```python
from build123d import *

# Parameters (mm, degrees)
SKETCH_1_W          = 15
SKETCH_1_H          = 15
EXTRUDE_1_DEPTH     = 5
SKETCH_2_R          = 1.25
SKETCH_2_R_2        = 2.8
SKETCH_2_R_3        = 1.5
SKETCH_2_R_4        = 1
CUT_EXTRUDE_1_DEPTH = 5
FILLET_1_R          = 1.5
SKETCH_4_R          = 1.5
EXTRUDE_2_DEPTH     = 2
SKETCH_5_R          = 2
CUT_EXTRUDE_2_DEPTH = 5


with BuildPart() as part:
    # 草图1 → 凸台-拉伸1 (new body)
    with BuildSketch(Plane(origin=(0, 0, 0), x_dir=(1, 0, 0), z_dir=(0, 1, 0))):
        Polygon((25, 10), (-25, 10), (-25, 5), (-25, -10), (25, -10), align=None)
        with Locations((-32.5, -2.5)):
            Rectangle(SKETCH_1_W, SKETCH_1_H)
    extrude(amount=EXTRUDE_1_DEPTH)

    # 草图2 → 切除-拉伸1 (cut)
    with BuildSketch(Plane(origin=(0, 5, 0), x_dir=(1, 0, 0), z_dir=(0, 1, 0))):
        with Locations(Location((0, 0, 0), (0, 0, 270))):
            Circle(SKETCH_2_R)
        with Locations(Location((15, 0, 0), (0, 0, 270))):
            Circle(SKETCH_2_R_2)
        with Locations(Location((-15, 0, 0), (0, 0, 270))):
            Circle(SKETCH_2_R_2)
        with Locations(Location((15, 8, 0), (0, 0, 270))):
            Circle(SKETCH_2_R)
        with Locations(Location((23, 0, 0), (0, 0, 270))):
            Circle(SKETCH_2_R)
        with Locations(Location((-23, 0, 0), (0, 0, 270))):
            Circle(SKETCH_2_R)
        with Locations(Location((-15, 8, 0), (0, 0, 270))):
            Circle(SKETCH_2_R)
        with Locations(Location((-32.5, -2.5, 0), (0, 0, 270))):
            Circle(SKETCH_2_R_3)
        with Locations(Location((-27, -2.5, 0), (0, 0, 270))):
            Circle(SKETCH_2_R_4)
        with Locations(Location((-32.5, -8, 0), (0, 0, 270))):
            Circle(SKETCH_2_R_4)
        with Locations(Location((-38, -2.5, 0), (0, 0, 270))):
            Circle(SKETCH_2_R_4)
        with Locations(Location((-32.5, 3, 0), (0, 0, 270))):
            Circle(SKETCH_2_R_4)
    extrude(amount=-CUT_EXTRUDE_1_DEPTH, mode=Mode.SUBTRACT)

    # 圆角1
    fillet_1_edges = [part.edges().sort_by_distance(p)[0] for p in [
        (-25, 2.5, -5),
        (-40, 2.5, -5),
        (-25, 2.5, -10),
        (25, 2.5, -10),
    ]]
    fillet(fillet_1_edges, radius=FILLET_1_R)

    # 草图4 → 凸台-拉伸2 (add)
    with BuildSketch(Plane.XY.offset(10)):
        with Locations(Location((20, 2.5, 0), (0, 0, 180))):
            Circle(SKETCH_4_R)
        with Locations(Location((-20, 2.5, 0), (0, 0, 180))):
            Circle(SKETCH_4_R)
    extrude(amount=EXTRUDE_2_DEPTH)

    # 草图5 → 切除-拉伸2 (cut)
    with BuildSketch(Plane(origin=(0, 0, -10), x_dir=(-1, 0, 0), z_dir=(0, 0, -1))):
        with Locations((-20, 2.5)):
            Circle(SKETCH_5_R)
        with Locations(Location((20, 2.5, 0), (0, 0, 180))):
            Circle(SKETCH_5_R)
    extrude(amount=-CUT_EXTRUDE_2_DEPTH, mode=Mode.SUBTRACT)


solid = part.part
```
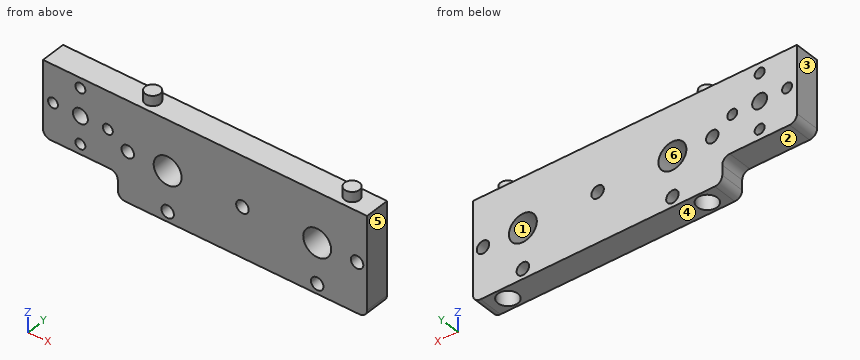
CAD build for the part. Positions are in the model's coordinates, mm. Face numbers are marked on the shaded views. A direction names the side the tool comes from. Give positions to 0.01 mm unless a question says otherwise; leave off trailing zeros. Order: outer loops, then holes, each group sorted by start corner. A loop starts at its lowest first (then second) coordinate and runs counter-clockwise, first axis right, second up. Notation, with made-up numbers: M 34,78.5 L 54,78.5 A26 cw 54,104.5 Z; hole C 53.25,81.25 d11. An arc over 180 degrees is marked long. Put each result on its own line as item: value. Start each with the question number.
(1) Drill centre lines: line 1 along X through (y, z) = (3.7, 0); line 2 along X through (y, z) = (3.35, 8); line 3 along Z through (x, y) = (-14, 3.55). Where is each one in solid material? Low to high.
(2) Saw through at A-A, the plane x = 0. Write the cut outline in (y, z), then the cut area to 3 significant figures.
(3) Which spindle directions (+Z, -Z, +X, -X, +Y, -Y) get a long thin tool onto all of the face, cutting with end or side? Do the marked faces 1 and 2. Say none if no direction does.
(4) Saw through at B-B, the plane z = 0. Write the cut outline in (x, y).
(5) Saw through at D-D, the plane z = 8. Write the cut outline in (x, y), then the cut area to 3 significant figures.
(6) Mould opens along X. For the marked faces 3, 4, 5 and 6 say: +X half, -X half, draft (parallel to the pull), parting line (faces both ways), or undercut.
(7) Saw through at C-C, the plane x = 15. Write the cut outline in (y, z).
(8) Flat gauge pins, fed straight in: pin 1 Ø1.5 at (x, y) = (-15, 3) entering from +Z; pin 2 Ø2 at (y, z) = (2.5, -7.5) entering from -X; pin 3 Ø1.6 at (x, z) = (-32.5, -3) entering from +Y; pin 4 Ø1.5 at (x, y) = (-31, 2) entering from -Z. Where does each tip first touch, or does it go through?
Check result:
1. line 1: x = -40 to -24.25, -21.75 to -17.8, -12.2 to -1.25, 1.25 to 12.2, 17.8 to 21.75, 24.25 to 25
1. line 2: x = -40 to -33.5, -31.5 to 25
1. line 3: z = -10 to -8.75, -7.25 to -2.62, 2.62 to 10
2. outline: M 0,-10 L 5,-10 L 5,-1.25 L 0,-1.25 Z; M 0,1.25 L 5,1.25 L 5,10 L 0,10 Z
2. area: 87.5 mm2
3. face 1: +Y, -Y
3. face 2: -Z, -X, +Y, -Y
4. outline: M -40,0 L -24.25,0 L -24.25,5 L -40,5 Z; M -21.75,0 L -17.8,0 L -17.8,5 L -21.75,5 Z; M -12.2,0 L -1.25,0 L -1.25,5 L -12.2,5 Z; M 1.25,0 L 12.2,0 L 12.2,5 L 1.25,5 Z; M 17.8,0 L 21.75,0 L 21.75,5 L 17.8,5 Z; M 24.25,0 L 25,0 L 25,5 L 24.25,5 Z
5. outline: M -40,0 L -33.5,0 L -33.5,5 L -40,5 Z; M -31.5,0 L 25,0 L 25,5 L -31.5,5 Z
5. area: 315 mm2
6. face 3: -X half
6. face 4: draft
6. face 5: +X half
6. face 6: undercut
7. outline: M 0,-10 L 5,-10 L 5,-9.25 L 0,-9.25 Z; M 0,-6.75 L 5,-6.75 L 5,-2.8 L 0,-2.8 Z; M 0,2.8 L 5,2.8 L 5,10 L 0,10 Z
8. pin 1: stops at z = 10
8. pin 2: stops at x = -25
8. pin 3: passes through
8. pin 4: stops at z = -5
